from build123d import *

# Parameters (mm, degrees)
SKETCH1_R           = 29
BOSS_EXTRUDE1_DEPTH = 8
SKETCH2_R           = 26
BOSS_EXTRUDE2_DEPTH = 11
SKETCH3_R           = 24.5
CUT_EXTRUDE1_DEPTH  = 3


with BuildPart() as part:
    # Sketch1 → Boss-Extrude1 (new body)
    with BuildSketch(Plane(origin=(0, 0, 0), x_dir=(1, 0, 0), z_dir=(0, 1, 0))):
        Circle(SKETCH1_R)
    extrude(amount=-BOSS_EXTRUDE1_DEPTH)

    # Sketch2 → Boss-Extrude2 (add)
    with BuildSketch(Plane.XZ.offset(8)):
        Circle(SKETCH2_R)
    extrude(amount=BOSS_EXTRUDE2_DEPTH)

    # Sketch3 → Cut-Extrude1 (cut)
    with BuildSketch(Plane(origin=(0, 0, 0), x_dir=(1, 0, 0), z_dir=(0, 1, 0))):
        Circle(SKETCH3_R)
    extrude(amount=-CUT_EXTRUDE1_DEPTH, mode=Mode.SUBTRACT)


solid = part.part
Source: CAD feature listing. Evaluate the final solid. Frame: model axes, mm. A direction names the side the tool comes from. Round coordinates to 2 decimals unless told otherwise and drop trailing zeros. Order: outer loops, then holes, each group sorted by start corner. A loop starts at its lowest first (then second) coordinate and runs counter-clockwise, first axis right, second up. Notation, with made-up numbers: (-28, 51.25) - (9, 51.25) arc R26 ccw to (9, 77.25) - close; hole circle Ø9 at (-18.5, 68). An arc over 180 degrees is marked (long way). Use a Markdown table: item, result. Add a question column.
1. Section query B-B (x = 0). Return the cut outline in (y, z).
2. Section query C-C (y = -1.5). Return the cut outline in (x, z).
3. Line query: probe 1 along Z at (x, y) = (0, -1.9); probe 2 along Y at (x, z) = (-7.5, 9). Output: solid intervals per line, ascending.
4. Section query D-D (y = -12.5). Return the cut outline in (x, z).
5. Section query A-A (z = 0). Return the cut outline in (x, y).
6. Set-up query: faces 1 (the cylindrical face through (13.38, -3.94, 25.73)), 2 (the flat face through (0, -3, 0)), 3 (the flat face through (-11, -8, -24)). Return all of +Z, -Z, +X, -X, +Y, -Y with unobstructed straight access to the full face (end or side cutting, diameter ignored); none if empty.
7. First-contact query: pin 1 (1.5 mm diameter, centred on y = -7.5, z = 14, fed in from -X); pin 2 (8 mm diameter, centred on x = 10, z = 5, fed in from +Y); pin 3 (4 mm diameter, centred on x = 8, y = -16.5, fed in from -Z); pin 4 (6 mm diameter, centred on x = -16, z = 23, fed in from +Y). Flat tips, straight axial feed; report the tip coordinate or a pass-through.
Derived:
| question | item | result |
|---|---|---|
| 1 | outline | (-19, -26) - (-8, -26) - (-8, -29) - (0, -29) - (0, -24.5) - (-3, -24.5) - (-3, 24.5) - (0, 24.5) - (0, 29) - (-8, 29) - (-8, 26) - (-19, 26) - close |
| 2 | outline | circle Ø58 at (0, 0); hole circle Ø49 at (0, 0) |
| 3 | probe 1 | -29 to -24.5, 24.5 to 29 |
| 3 | probe 2 | -19 to -3 |
| 4 | outline | circle Ø52 at (0, 0) |
| 5 | outline | (-29, -8) - (-26, -8) - (-26, -19) - (26, -19) - (26, -8) - (29, -8) - (29, 0) - (24.5, 0) - (24.5, -3) - (-24.5, -3) - (-24.5, 0) - (-29, 0) - close |
| 6 | face 1 | +Y, -Y |
| 6 | face 2 | +Y |
| 6 | face 3 | -Y |
| 7 | pin 1 | x = -25.8 |
| 7 | pin 2 | y = -3 |
| 7 | pin 3 | z = -25.3 |
| 7 | pin 4 | y = 0 |
